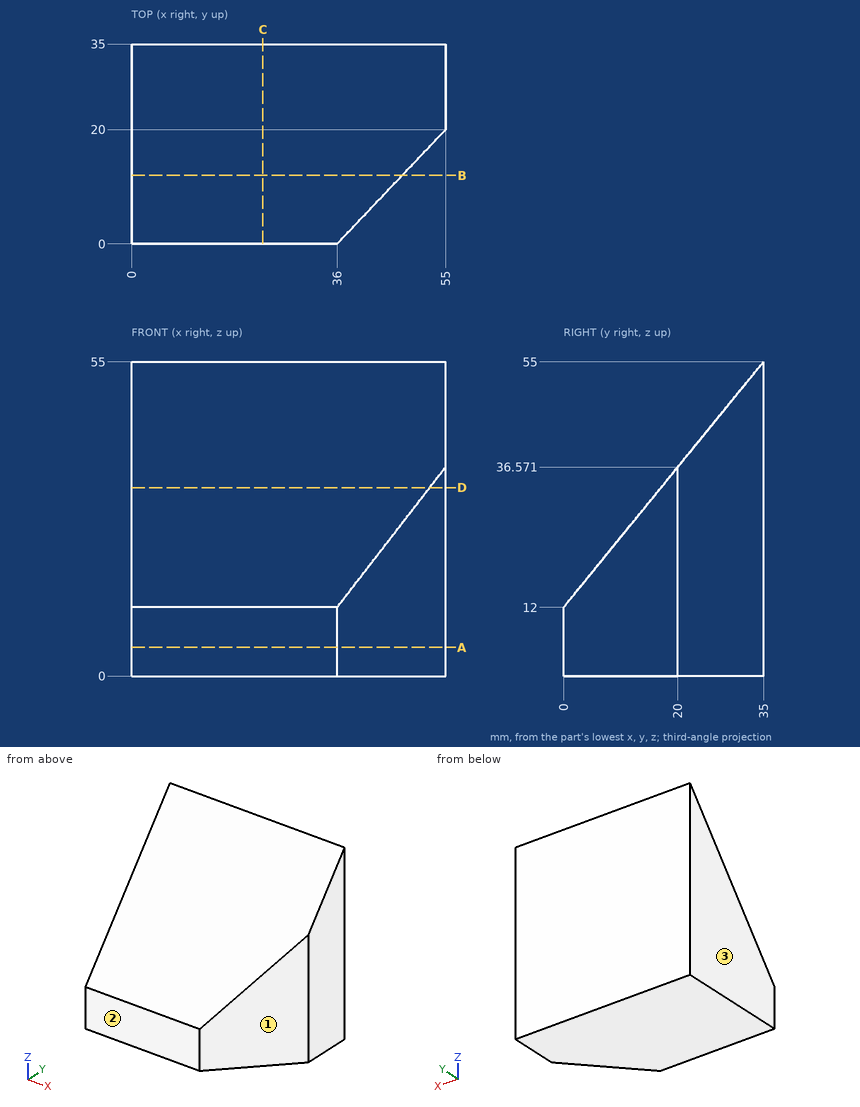
Verification items for this drawing (mm, ordinates from the low corner). Round coordinates to 2 decimals unless told otherwise and drop trailing zeros. Order: outer loops, then holes, each group sorted by start corner. A loop starts at its lowest first (then second) coordinate and runs counter-clockwise, first axis right, second up. Notation, with made-up numbers: (35.5, 8.25) - (60.5, 8.25) arc R28 ccw to (60.5, 35.25) - close; hole circle Ø8 at (-13.75, 58). An arc over 180 degrees is marked (long way). Answer as CSV lines item,"result". Start each with the question number.
1) Draft check along X on the marked faces 1, 2 and 3. Enter one of: +X half, -X half, draft (parallel to the pull), parting line (faces both ways), or undercut.
2) Section check B-B (y = 12). Record the cut outline in (x, z), then the cut area to 3 significant figures.
3) Section check C-C (x = 23). Record the cut outline in (y, z).
4) Scan lines: probe 1 along Y at (x, z) = (42, 25); probe 2 along Z at (x, y) = (25, 16.5); probe 3 along Y at (x, z) = (45, 22.5) (1 decimal). Record each from-to range of solid material in increasing order.
5) Section check D-D (z = 33). Record the cut outline in (x, y), then the cut area to 3 significant figures.
6) Depth check by flat-ended pin: pin 1 (1 mm diameter, centred on x = 33.5, y = 11, fed in from +Z); pin 2 (1.5 mm diameter, centred on y = 29, z = 41, fed in from -X); pin 3 (2 mm diameter, centred on x = 44.5, y = 13, fed in from +Z); pin 4 (12 mm diameter, centred on x = 35.5, y = 8.5, fed in from +Z) (1 decimal). Enter the tip coordinate at first touch or a pass-through.
7) Section check A-A (z = 5). Record the cut outline in (x, y).
Determined:
1,face 1,"+X half"
1,face 2,"draft"
1,face 3,"-X half"
2,outline,"(0, 0) - (47.4, 0) - (47.4, 26.74) - (0, 26.74) - close"
2,area,"1,270 mm^2"
3,outline,"(0, 0) - (35, 0) - (35, 55) - (0, 12) - close"
4,probe 1,"10.58 to 35"
4,probe 2,"0 to 32.27"
4,probe 3,"9.5 to 35"
5,outline,"(0, 17.09) - (52.24, 17.09) - (55, 20) - (55, 35) - (0, 35) - close"
5,area,"981 mm^2"
6,pin 1,"z = 26.13"
6,pin 2,"x = 0"
6,pin 3,"z = 29.2"
6,pin 4,"z = 29.8"
7,outline,"(0, 0) - (36, 0) - (55, 20) - (55, 35) - (0, 35) - close"
